Here's how the part is built. I have some questions about the finished solid (model axes, mm). Face numbers are marked on the shaded views. A direction names the side the tool comes from. Give positions to 0.01 mm unless a question says otherwise; leave off trailing zeros. Order: outer loops, then holes, each group sorted by start corner. A loop starts at its lowest first (then second) coordinate and runs counter-clockwise, first axis right, second up. Notation, with made-up numbers: (-13.75, 53) - (45.25, 53) arc R22 cw to (45.25, 73) - close; hole circle Ø5 at (79.25, -35.75). An arc over 180 degrees is marked (long way). One line per question, with ' | ' between items.
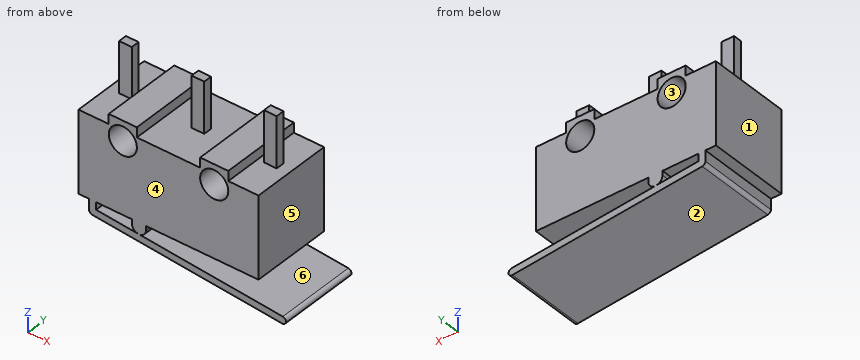
from build123d import *

# Parameters (mm, degrees)
SKETCH1_R           = 1
BOSS_EXTRUDE1_DEPTH = 5.8
SKETCH3_W           = 0.9
SKETCH3_H           = 0.6
BOSS_EXTRUDE2_DEPTH = 3.6


with BuildPart() as part:
    # Sketch1 → Boss-Extrude1 (new body)
    with BuildSketch(Plane(origin=(0, 0, 0), x_dir=(1, 0, 0), z_dir=(0, 1, 0))):
        with BuildLine():
            ThreePointArc((-1.6, 3.2), (-1.7066364, 3.508650414), (-1.981060312, 3.685647352))
            Line((-1.981060312, 3.685647352), (-1.981060312, 3.713031937))
            Line((-1.981060312, 3.713031937), (8.122870222, 4.641240594))
            ThreePointArc((8.122870222, 4.641240594), (8.348951708, 4.913062524), (8.077129778, 5.13914401))
            Line((8.077129778, 5.13914401), (-5.422870222, 3.898951708))
            ThreePointArc((-5.422870222, 3.898951708), (-5.584685619, 3.81849695), (-5.65, 3.65))
            Line((-5.65, 3.65), (-5.65, 2.9))
            Line((-5.65, 2.9), (-6.4, 2.9))
            Line((-6.4, 2.9), (-6.4, -2.9))
            Line((-6.4, -2.9), (-4.25, -2.9))
            Line((-4.25, -2.9), (-4.25, -3.6))
            Line((-4.25, -3.6), (-2.25, -3.6))
            Line((-2.25, -3.6), (-2.25, -2.9))
            Line((-2.25, -2.9), (2.25, -2.9))
            Line((2.25, -2.9), (2.25, -3.6))
            Line((2.25, -3.6), (4.25, -3.6))
            Line((4.25, -3.6), (4.25, -2.9))
            Line((4.25, -2.9), (6.4, -2.9))
            Line((6.4, -2.9), (6.4, 2.9))
            Line((6.4, 2.9), (-1.6, 2.9))
            Line((-1.6, 2.9), (-1.6, 3.2))
        make_face()
        with Locations(Location((-3.25, -2.2, 0), (0, 0, 270))):
            Circle(SKETCH1_R, mode=Mode.SUBTRACT)
        with Locations(Location((3.25, -2.2, 0), (0, 0, 270))):
            Circle(SKETCH1_R, mode=Mode.SUBTRACT)
        with BuildLine():
            Line((-2.218939688, 3.691178887), (-2.218939688, 3.685647352))
            ThreePointArc((-2.218939688, 3.685647352), (-2.4933636, 3.508650414), (-2.6, 3.2))
            Line((-2.6, 3.2), (-2.6, 2.9))
            Line((-2.6, 2.9), (-5.15, 2.9))
            Line((-5.15, 2.9), (-5.15, 3.421913818))
            Line((-5.15, 3.421913818), (-2.218939688, 3.691178887))
        make_face(mode=Mode.SUBTRACT)
    extrude(amount=BOSS_EXTRUDE1_DEPTH)

    # Sketch3 → Boss-Extrude2 (add)
    with BuildSketch(Plane.XY.offset(2.9)):
        with Locations((-5.15, 2.9)):
            Rectangle(SKETCH3_W, SKETCH3_H)
        with Locations((0, 2.9)):
            Rectangle(SKETCH3_W, SKETCH3_H)
        with Locations((5.15, 2.9)):
            Rectangle(SKETCH3_W, SKETCH3_H)
    extrude(amount=BOSS_EXTRUDE2_DEPTH)


solid = part.part
1) I want a section at B-B (x = -3.25). List the corners of the cut face in (y, z) for me.
Model answer:
outline: (0, -4.1) - (5.8, -4.1) - (5.8, -3.6) - (0, -3.6) - close; (0, -2.9) - (5.8, -2.9) - (5.8, 1.2) - (0, 1.2) - close; (0, 3.2) - (5.8, 3.2) - (5.8, 3.6) - (0, 3.6) - close
2) On a 3-axis mill with a long thin cutter (end or side, diameter ignored), from which of +Z, -Z, +X, -X, +Y, -Y can I reach the whole of each face in a straight line? I mean the marked faces 4, 5 and 6. Say none if no direction works.
Model answer:
face 4: +Z, -Z, +X, -X, -Y | face 5: +Z, +X, +Y, -Y | face 6: +X, +Y, -Y
3) Thinking about a two-plate mould opening in Z: for the marked faces 1, 2 and 3, which applies, +Z half, -Z half, draft (parallel to the pull), parting line (faces both ways), or undercut?
Model answer:
face 1: draft | face 2: -Z half | face 3: undercut
4) I want a section at A-A (y = 4.55). State how many separate pieces and enclosed holes the cut face has, plus the area to 3 significant figures.
Model answer:
separate pieces: 1 | enclosed holes: 3 | area: 78.7 mm2
5) Please list where these lines run through material, in increasing order: L1, parallel to X at y = 1.55, z = 2.2; L2, parallel to Z at x = 2.75, y = 2.5; L3, parallel to X at y = 2.5, z = 3.
Model answer:
L1: x = -6.4 to -4.25, -2.25 to 2.25, 4.25 to 6.4 | L2: z = -4.65 to -4.15, -2.9 to 1.33, 3.07 to 3.6 | L3: x = -4.25 to -3.85, -2.65 to -2.25, 2.25 to 2.65, 3.85 to 4.25
6) I want a section at C-C (x = 1). List the corners of the cut face in (y, z) for me, plus the area to 3 significant figures.
Model answer:
outline: (0, -4.49) - (5.8, -4.49) - (5.8, -3.99) - (0, -3.99) - close; (0, -2.9) - (5.8, -2.9) - (5.8, 2.9) - (0, 2.9) - close | area: 36.6 mm2
7) I want a section at D-D (z = 0). List the corners of the cut face in (x, y) for me, plus the area to 3 significant figures.
Model answer:
outline: (-6.4, 0) - (6.4, 0) - (6.4, 5.8) - (-6.4, 5.8) - close | area: 74.2 mm2
8) I'm going to push flat-ended pins straight in: P1, Ø1.5, axis at y = 5, z = 4.5, coming from the +X side; P2, Ø1, axis at x = 0, z = 4, coming from the +Y side; P3, Ø0.7, axis at y = 3, z = 4, coming from the -X side; P4, Ø0.8, axis at x = -3.5, y = 1.5, coming from the -Z side. Where does each tip first touch, or does it pass through?
Model answer:
P1: passes through | P2: stops at y = 3.2 | P3: stops at x = -5.6 | P4: stops at z = -4.11
